The listing builds one solid part. Answer for the finished solid, in the listing's coordinates (mm). A direction names the side the tool comes from. Round coordinates to 2 decimals unless told otherwise and drop trailing zeros. Loops run counter-clockwise (first coordinate to the right, second up) from the corner with the lowest first, then second, coordinate; pieces in that order, holes last. Notation, with made-up numbers: (18, -23.75) -> (69, -23.75) arc R24 cw to (69, 14.25) -> close; hole circle Ø6 at (65, 17.5). An arc over 180 degrees is marked (long way). Use a Markdown table: item, result. Add a question column.
Q1. Consider line 1 (X direction, y = -0.75, z = 1.8); line 2 (Y direction, x = 1.5, z = 0.35); line 3 (X direction, y = 0.5, z = 1.2). Determine where each line is inside the solid, lowest interval first.
Q2. For a pull along X with two mould halves and no side action, classify faces 1 (the flat face through (-6, 6, 1)), 2 (the flat face through (0, 9, 1)), 3 (the flat face through (1, 12, 1)), 4 (the flat face through (-2, 6, 1)) as released by +X, released by -X, zero draft, split by the parting line, or undercut.
Q3. Section C-C on y = 11 is taken. Give the vertices of the cut face in (x, z), then the cut area to 3 significant figures.
Q4. Given pin 1 Ø1.5 at (x, z) = (-1.5, 1.5) entering from +Y; pin 2 Ø1.5 at (y, z) = (-1, 1.5) entering from -X; pin 3 Ø1.5 at (y, z) = (2, 2) entering from -X, each flat-ended and moving along its own axis, determine where each tip first touches the part or whether it passes through.
Q5. Section A-A on z = 1.95 is taken. Give the vertices of the cut face in (x, y), then the cut area to 3 significant figures.
Q6. Section B-B on y = 7.75 is taken. Give the vertices of the cut face in (x, z) (3 decimals).
Q7. Section D-D on x = -1.5 is taken. Give the vertices of the cut face in (y, z).
Q8. Which of the six approach directions +Z, -Z, +X, -X, +Y, -Y give full straight-line access (tool end or side, diameter ignored) to faces 5 (the flat face through (60, 3, 1)), 6 (the flat face through (13, -3, 1)), 7 (the flat face through (5, -2, 1)), 8 (the flat face through (29, 0, 1)), 9 (the flat face through (53, -1, 1))?
Autodesk Inventor part; units mm, degrees
ref_plane "YZ Plane" through (0, 0, 0) normal (1, 0, 0) x (0, 1, 0)
ref_plane "XZ Plane" through (0, 0, 0) normal (0, 1, 0) x (-1, 0, 0)
ref_plane "XY Plane" through (0, 0, 0) normal (0, 0, 1) x (1, 0, 0)
sketch "Sketch1" plane through (0, 0, 0) normal (0, 0, 1) x (1, 0, 0)
  line L0 (0, 0) -> (0, 12)
  line L1 (60, 6) -> (60, 0)
  line L2 (60, 0) -> (0, 0)
  line L3 (0, 3) -> (-6, 3)
  line L4 (-6, 3) -> (-6, 9)
  line L5 (-6, 9) -> (-3, 9)
  line L6 (-3, 9) -> (-3, 6)
  line L7 (-3, 6) -> (0, 6)
  line L8 (5, 0) -> (21, 0)
  line L9 (21, 0) -> (21, -3)
  line L10 (21, -3) -> (5, -3)
  line L11 (5, -3) -> (5, 0)
  line L12 (37, 0) -> (53, 0)
  line L13 (53, 0) -> (53, -3)
  line L14 (53, -3) -> (37, -3)
  line L15 (37, -3) -> (37, 0)
  line L16 (0, 12) -> (3, 12)
  line L17 (3, 12) -> (60, 6)
  dimension "d0" = 3
  dimension "d1" = 3
  dimension "d2" = 3
  dimension "d3" = 3
  dimension "d4" = 3
  dimension "d5" = 3
  dimension "d6" = 16
  dimension "d7" = 5
  dimension "d8" = 16
  dimension "d9" = 7
  dimension "d10" = 3
  dimension "d11" = 6
  dimension "d12" = 3
extrude "Extrusion1" add sketch "Sketch1" along normal blind 3
equation "\"BendRadius\" = Thickness"
equation "\"BendReliefWidth\" = Thickness"
equation "\"BendReliefDepth\" = 0.5 * Thickness"
equation "\"CornerReliefSize\" = 4 * Thickness"
equation "\"MinimumRemnant\" = 2 * Thickness"
equation "\"TransitionRadius\" = BendRadius"
equation "\"JacobiRadiusSize\" = BendRadius"
equation "\"GapSize\" = Thickness"
properties part number "tail fin" material "Hardboard"
Checked values:
| question | item | result |
|---|---|---|
| 1 | line 1 | x = 5 to 21, 37 to 53 |
| 1 | line 2 | y = 0 to 12 |
| 1 | line 3 | x = 0 to 60 |
| 2 | face 1 | released by -X |
| 2 | face 2 | undercut |
| 2 | face 3 | zero draft |
| 2 | face 4 | undercut |
| 3 | outline | (0, 0) -> (12.5, 0) -> (12.5, 3) -> (0, 3) -> close |
| 3 | area | 37.5 mm2 |
| 4 | pin 1 | stops at y = 6 |
| 4 | pin 2 | stops at x = 5 |
| 4 | pin 3 | stops at x = 0 |
| 5 | outline | (-6, 3) -> (0, 3) -> (0, 0) -> (5, 0) -> (5, -3) -> (21, -3) -> (21, 0) -> (37, 0) -> (37, -3) -> (53, -3) -> (53, 0) -> (60, 0) -> (60, 6) -> (3, 12) -> (0, 12) -> (0, 6) -> (-3, 6) -> (-3, 9) -> (-6, 9) -> close |
| 5 | area | 672 mm2 |
| 6 | outline | (-6, 0) -> (-3, 0) -> (-3, 3) -> (-6, 3) -> close; (0, 0) -> (43.375, 0) -> (43.375, 3) -> (0, 3) -> close |
| 7 | outline | (3, 0) -> (6, 0) -> (6, 3) -> (3, 3) -> close |
| 8 | face 5 | +Z, -Z, +X, +Y, -Y |
| 8 | face 6 | +Z, -Z, +X, -X, -Y |
| 8 | face 7 | +Z, -Z, -X, -Y |
| 8 | face 8 | +Z, -Z, -Y |
| 8 | face 9 | +Z, -Z, +X, -Y |
